The listing builds one solid part. Answer for the finished solid, in the listing's coordinates (mm). A direction names the side the tool comes from. Coordinates: 2 decimals unless noted, no trailing zeros. Order: outer loops, then holes, each group sorted by start corner. A loop starts at its lowest first (then second) coordinate and runs counter-clockwise, first axis right, second up. Notation, with made-up numbers: (3.25, 35) - (9.25, 35) arc R20 cw to (9.25, 67) - close; hole circle Ø8 at (26.25, -21). An arc over 180 degrees is marked (long way). Use one line per item in the form item = value. Start each with the question number.
Item 1: Section A-A, the plane x = -14 is taken. Write down the section's boundary in (y, z), and give its area (3 significant figures).
Item 2: Section D-D, the plane z = 53.5 is taken. Write down the section's boundary in (x, y), and give its area (3 significant figures).
Item 3: Section C-C, the plane y = 103 is taken. Write down the section's boundary in (x, z).
Item 4: Each of these flat-tipped pins is pushed along its axis until it touches: pin 1 Ø4.5 at (x, y) = (16, -102) entering from +Z; pin 2 Ø12 at (y, z) = (96.5, 87) entering from +X; pin 3 Ø24 at (x, y) = (77.5, -103) entering from +Z. Where does it stop, or does it pass through?
Item 5: A tool of negligible diameter and unlimited length cuts with its end or side. For faces 4 (the flat face through (17, -105, 90)), 5 (the flat face through (-125, -1, 28)), 6 (the flat face through (-95, -105, 65)), from which of +Z, -Z, +X, -X, +Y, -Y can it reach the whole face along a straight path? Write none if from no direction.
Item 6: Consider line 1 along Y through (x, z) = (106.5, 37.5); line 2 along Y through (x, z) = (-32.5, 48); line 3 along X through (y, z) = (112.5, 99.5). Determine where each line is inside the solid, lowest interval first. Write a range as [from, to].
Item 7: The mould has two halves that part along Y. Classify faces 1 (the flat face through (-6, 85, 49)), 2 (the flat face through (-2, -125, 34)), 3 (the flat face through (-15, -105, 75)): released by +Y, released by -Y, zero draft, split by the parting line, or undercut.
Item 8: Section B-B, the plane z = 80 is taken. Write down the section's boundary in (x, y), and give its area (3 significant figures).
from build123d import *

# Parameters (mm, degrees)
F0_W      = 350
F0_H      = 250
F1_DEPTH  = 40
F2_W      = 170
F2_H      = 25
F3_DEPTH  = 300
F4_W      = 150
F4_H      = 10
F5_DEPTH  = 25
F6_W      = 120
F6_H      = 40
F7_DEPTH  = 50
F8_W      = 120
F8_H      = 40
F9_DEPTH  = 65
F10_W     = 50
F10_H     = 15
F11_DEPTH = 250.001


with BuildPart() as f1:
    # F0 (on Top) → F1 (new body)
    with BuildSketch(Plane.XY):
        Rectangle(F0_W, F0_H)
    extrude(amount=F1_DEPTH)

    # F2 (on face) → F3 (cut)
    with BuildSketch(Plane.YZ.offset(175)):
        with Locations((0, 27.5)):
            Rectangle(F2_W, F2_H)
    extrude(amount=-F3_DEPTH, mode=Mode.SUBTRACT)

    # F4 (on face) → F5 (cut)
    with BuildSketch(Plane.XY.offset(40)):
        with Locations((100, -90)):
            Rectangle(F4_W, F4_H)
    extrude(amount=-F5_DEPTH, mode=Mode.SUBTRACT)

    # F6 (on face) → F7 (join)
    with BuildSketch(Plane.XY.offset(40)):
        with Locations((-35, -105)):
            Rectangle(F6_W, F6_H)
    extrude(amount=F7_DEPTH)

    # F8 (on face) → F9 (join)
    with BuildSketch(Plane.XY.offset(40)):
        with Locations((-15, 105)):
            Rectangle(F8_W, F8_H)
    extrude(amount=F9_DEPTH)

    # F10 (on face) → F11 (cut, through all)
    with BuildSketch(Plane.XZ.offset(125)):
        with Locations((-15, 82.5)):
            Rectangle(F10_W, F10_H)
    extrude(amount=-F11_DEPTH, mode=Mode.SUBTRACT)


solid = f1.part
Response:
q1.outline = (-125, 0) - (125, 0) - (125, 75) - (85, 75) - (85, 15) - (-85, 15) - (-85, 75) - (-125, 75) - close; (85, 90) - (125, 90) - (125, 105) - (85, 105) - close
q1.area = 9,150 mm2
q2.outline = (-95, -125) - (25, -125) - (25, -85) - (-95, -85) - close; (-75, 85) - (45, 85) - (45, 125) - (-75, 125) - close
q2.area = 9,600 mm2
q3.outline = (-175, 0) - (175, 0) - (175, 40) - (45, 40) - (45, 105) - (-75, 105) - (-75, 40) - (-175, 40) - close; hole (-40, 75) - (10, 75) - (10, 90) - (-40, 90) - close
q4.pin_1 = 90
q4.pin_2 = 45
q4.pin_3 = 40
q5.face_4 = +Z, +X, -X, -Y
q5.face_5 = +Z, +X
q5.face_6 = +Z, -X, +Y, -Y
q6.line_1 = [-125, -95], [85, 125]
q6.line_2 = [-125, -85], [85, 125]
q6.line_3 = [-75, 45]
q7.face_1 = undercut
q7.face_2 = released by -Y
q7.face_3 = zero draft
q8.outline = (-95, -125) - (-40, -125) - (-40, -85) - (-95, -85) - close; (-75, 85) - (-40, 85) - (-40, 125) - (-75, 125) - close; (10, -125) - (25, -125) - (25, -85) - (10, -85) - close; (10, 85) - (45, 85) - (45, 125) - (10, 125) - close
q8.area = 5,600 mm2
